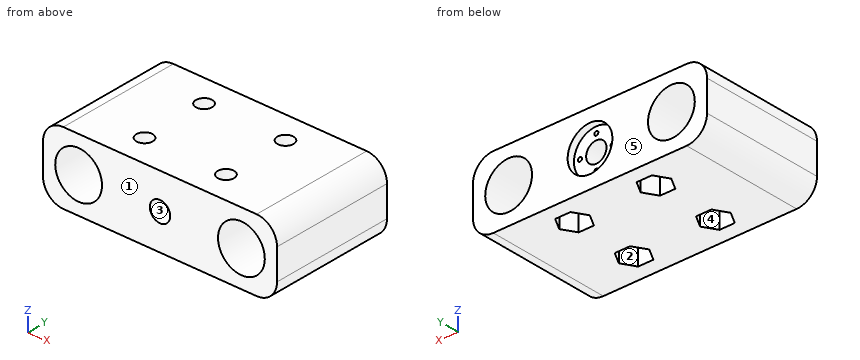
from build123d import *

# Parameters (mm, degrees)
SKETCH1_R           = 11.5
SKETCH1_R_2         = 5
BOSS_EXTRUDE1_DEPTH = 61
SKETCH2_R           = 11
SKETCH2_R_2         = 1
CUT_EXTRUDE1_DEPTH  = 3.5
SKETCH2_2_R         = 1
CUT_EXTRUDE2_DEPTH  = 13.5
SKETCH4_R           = 4
CUT_EXTRUDE3_DEPTH  = 135.799851632
CUT_EXTRUDE4_START  = -25
SKETCH4_3_R         = 4
CUT_EXTRUDE4_DEPTH  = 10


with BuildPart() as part:
    # Sketch1 → Boss-Extrude1 (new body)
    with BuildSketch(Plane(origin=(0, 0, 0), x_dir=(1, 0, 0), z_dir=(0, 1, 0))):
        with BuildLine():
            Line((10, 0), (105, 0))
            ThreePointArc((105, 0), (112.071067812, 2.928932188), (115, 10))
            Line((115, 10), (115, 25))
            ThreePointArc((115, 25), (112.071067812, 32.071067812), (105, 35))
            Line((105, 35), (10, 35))
            ThreePointArc((10, 35), (2.928932188, 32.071067812), (0, 25))
            Line((0, 25), (0, 10))
            ThreePointArc((0, 10), (2.928932188, 2.928932188), (10, 0))
        make_face()
        with Locations(Location((17.5, 17.5, 0), (0, 0, 90))):
            Circle(SKETCH1_R, mode=Mode.SUBTRACT)
        with Locations(Location((57.5, 17.5, 0), (0, 0, 90))):
            Circle(SKETCH1_R_2, mode=Mode.SUBTRACT)
        with Locations(Location((97.5, 17.5, 0), (0, 0, 90))):
            Circle(SKETCH1_R, mode=Mode.SUBTRACT)
    extrude(amount=BOSS_EXTRUDE1_DEPTH)

    # Sketch2 → Cut-Extrude1 (cut)
    with BuildSketch(Plane(origin=(0, 61, 0), x_dir=(1, 0, 0), z_dir=(0, 1, 0))):
        with Locations(Location((57.5, 17.5, 0), (0, 0, 270))):
            Circle(SKETCH2_R)
        with Locations(Location((57.5, 25.5, 0), (0, 0, 270))):
            Circle(SKETCH2_R_2, mode=Mode.SUBTRACT)
        with Locations(Location((65.5, 17.5, 0), (0, 0, 270))):
            Circle(SKETCH2_R_2, mode=Mode.SUBTRACT)
        with Locations(Location((57.5, 9.5, 0), (0, 0, 270))):
            Circle(SKETCH2_R_2, mode=Mode.SUBTRACT)
        with Locations(Location((49.5, 17.5, 0), (0, 0, 270))):
            Circle(SKETCH2_R_2, mode=Mode.SUBTRACT)
    extrude(amount=-CUT_EXTRUDE1_DEPTH, mode=Mode.SUBTRACT)

    # Sketch2<2> → Cut-Extrude2 (cut)
    with BuildSketch(Plane(origin=(0, 61, 0), x_dir=(1, 0, 0), z_dir=(0, 1, 0))):
        with Locations(Location((57.5, 25.5, 0), (0, 0, 270))):
            Circle(SKETCH2_2_R)
        with Locations(Location((65.5, 17.5, 0), (0, 0, 270))):
            Circle(SKETCH2_2_R)
        with Locations(Location((57.5, 9.5, 0), (0, 0, 270))):
            Circle(SKETCH2_2_R)
        with Locations(Location((49.5, 17.5, 0), (0, 0, 270))):
            Circle(SKETCH2_2_R)
    extrude(amount=-CUT_EXTRUDE2_DEPTH, mode=Mode.SUBTRACT)

    # Sketch4 → Cut-Extrude3 (cut, through all)
    with BuildSketch(Plane.XY):
        with Locations((37.5, 47)):
            Circle(SKETCH4_R)
        with Locations((37.5, 14)):
            Circle(SKETCH4_R)
        with Locations(Location((77.5, 14, 0), (0, 0, 180))):
            Circle(SKETCH4_R)
        with Locations(Location((77.5, 47, 0), (0, 0, 180))):
            Circle(SKETCH4_R)
    extrude(amount=-CUT_EXTRUDE3_DEPTH, mode=Mode.SUBTRACT)

    # Sketch4<3> → Cut-Extrude4 (cut)
    # profile 1 of 4: a face of its own
    with BuildSketch(Plane.XY.offset(CUT_EXTRUDE4_START)):
        Polygon((81.25277675, 20.5), (85.005553499, 14), (81.25277675, 7.5), (73.74722325, 7.5), (69.994446501, 14), (73.74722325, 20.5), align=None)
        with Locations((77.5, 14)):
            Circle(SKETCH4_3_R, mode=Mode.SUBTRACT)
    # profile 2 of 4: a face of its own
    with BuildSketch(Plane.XY.offset(CUT_EXTRUDE4_START)):
        Polygon((29.994446501, 47), (33.74722325, 40.5), (41.25277675, 40.5), (45.005553499, 47), (41.25277675, 53.5), (33.74722325, 53.5), align=None)
        with Locations((37.5, 47)):
            Circle(SKETCH4_3_R, mode=Mode.SUBTRACT)
    # profile 3 of 4: a face of its own
    with BuildSketch(Plane.XY.offset(CUT_EXTRUDE4_START)):
        Polygon((29.994446501, 14), (33.74722325, 7.5), (41.25277675, 7.5), (45.005553499, 14), (41.25277675, 20.5), (33.74722325, 20.5), align=None)
        with Locations((37.5, 14)):
            Circle(SKETCH4_3_R, mode=Mode.SUBTRACT)
    # profile 4 of 4: a face of its own
    with BuildSketch(Plane.XY.offset(CUT_EXTRUDE4_START)):
        Polygon((81.25277675, 53.5), (85.005553499, 47), (81.25277675, 40.5), (73.74722325, 40.5), (69.994446501, 47), (73.74722325, 53.5), align=None)
        with Locations((77.5, 47)):
            Circle(SKETCH4_3_R, mode=Mode.SUBTRACT)
    extrude(amount=-CUT_EXTRUDE4_DEPTH, mode=Mode.SUBTRACT)


solid = part.part
Geometry check sheet. Reference: the model listing, model coordinates, mm. Face numbers are marked on the shaded views. A direction names the side the tool comes from. Coordinates: 2 decimals unless noted, no trailing zeros. Write each loop counter-clockwise with the first axis right and the second up, starting at its lowest first coordinate (ties: lowest second). Pieces come first, ordered by that corner, then holes. Notation, with made-up numbers: (-18, -29.5) -> (-4, -29.5) arc R13 ccw to (-4, -9.5) -> close; hole circle Ø7 at (71.25, -32). An arc over 180 degrees is marked (long way). One line per question, with ' | ' between items.
1. Cross-section at A-A on z = -21. Record the cut outline in (x, y).
Answers:
outline: (0, 0) -> (6.55, 0) -> (6.55, 61) -> (0, 61) -> close; (28.45, 0) -> (53.93, 0) -> (53.93, 57.5) -> (47.07, 57.5) -> (47.07, 61) -> (28.45, 61) -> close; (61.07, 0) -> (86.55, 0) -> (86.55, 61) -> (67.93, 61) -> (67.93, 57.5) -> (61.07, 57.5) -> close; (108.45, 0) -> (115, 0) -> (115, 61) -> (108.45, 61) -> close; hole circle Ø8 at (37.5, 14); hole circle Ø8 at (37.5, 47); hole circle Ø8 at (77.5, 14); hole circle Ø8 at (77.5, 47)
2. Draft check along Y on the marked faces 1, 2 and 3. Enter one of: +Y half, -Y half, draft (parallel to the pull), parting line (faces both ways), or undercut.
Answers:
face 1: -Y half | face 2: undercut | face 3: draft
3. Depth check by flat-ended pin: pin 1 Ø7 at (x, y) = (77.5, 14) entering from +Z; pin 2 Ø6 at (y, z) = (28, -5.5) entering from -X; pin 3 Ø2 at (x, z) = (57.5, -10) entering from +Y; pin 4 Ø6.5 at (x, y) = (38, 46) entering from -Z. Enter the tip coordinate at first touch or a pass-through.
Answers:
pin 1: passes through | pin 2: stops at x = 0.11 | pin 3: stops at y = 57.5 | pin 4: stops at z = -25
4. Set-up check for the marked faces 4 and 5: record each of +Z, -Z, +X, -X, +Y, -Y from which the full face is reachable in a straight line by a thin tool's end or side.
Answers:
face 4: -Z | face 5: +Z, -Z, +X, -X, +Y
5. Cross-section at B-B on x = 17.5. Record the cut outline in (y, z).
Answers:
outline: (0, -35) -> (61, -35) -> (61, -29) -> (0, -29) -> close; (0, -6) -> (61, -6) -> (61, 0) -> (0, 0) -> close
6. Cross-section at C-C on y = 39. Record the cut outline in (x, z).
Answers:
outline: (0, -25) arc R10 ccw to (10, -35) -> (105, -35) arc R10 ccw to (115, -25) -> (115, -10) arc R10 ccw to (105, 0) -> (10, 0) arc R10 ccw to (0, -10) -> close; hole circle Ø23 at (17.5, -17.5); hole circle Ø10 at (57.5, -17.5); hole circle Ø23 at (97.5, -17.5)
7. Thickness scan on probe 1 along X at (y, z) = (25.5, -17.5); probe 2 along X at (y, z) = (17, -12); probe 3 along X at (y, z) = (40, -24). Record the ranges inside material, lowest first. Write a range as from..to.
Answers:
probe 1: x = 0..6, 29..52.5, 62.5..86, 109..115 | probe 2: x = 0..7.4, 27.6..34.85, 40.15..74.85, 80.15..87.4, 107.6..115 | probe 3: x = 0..8.01, 26.99..88.01, 106.99..115
8. Cross-section at D-D on z = -3. Record the cut outline in (x, y).
Answers:
outline: (2.86, 0) -> (112.14, 0) -> (112.14, 61) -> (2.86, 61) -> close; hole circle Ø8 at (37.5, 14); hole circle Ø8 at (37.5, 47); hole circle Ø8 at (77.5, 14); hole circle Ø8 at (77.5, 47)
